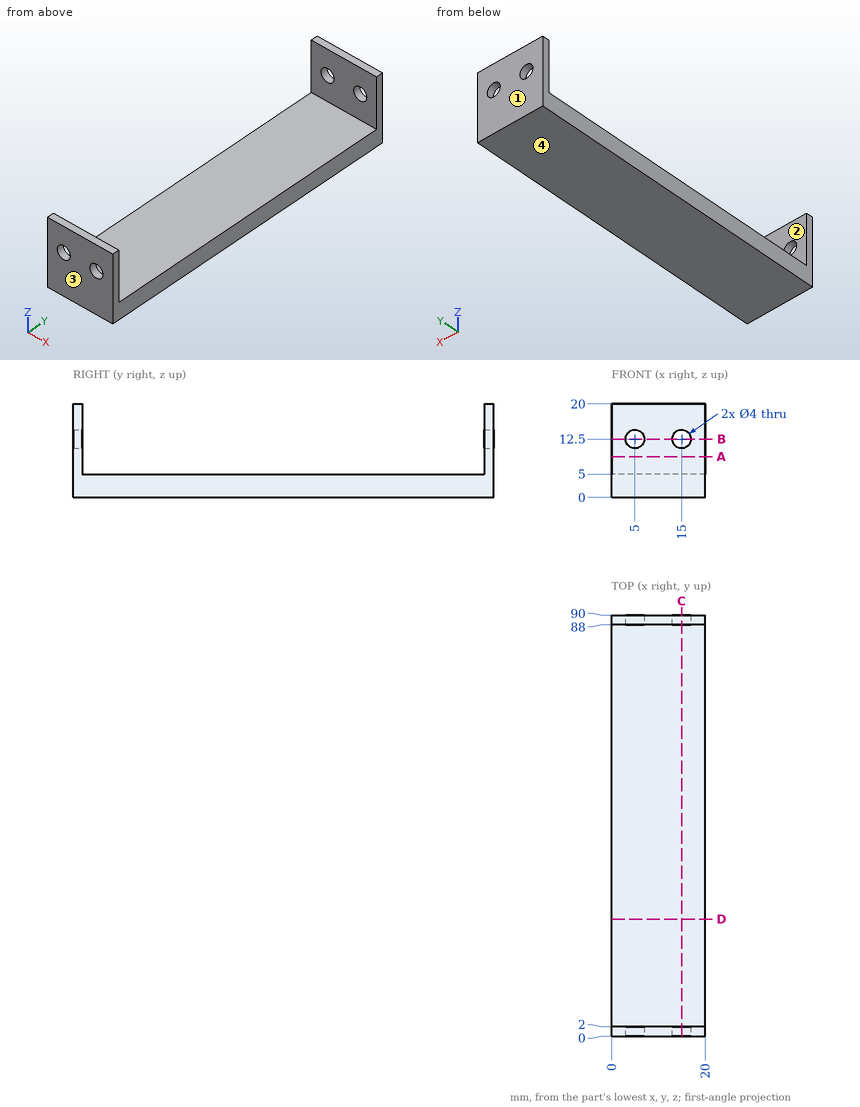
Job drawing, mm, ordinate dimensions from the low corner. One solid piece. Give positions to 0.01 mm unless a question says otherwise; leave off trailing zeros. Write each loop counter-clockwise with the first axis right and the second up, starting at its lowest first coordinate (ties: lowest second). Pieces come first, ordered by that corner, then holes. Notation, with made-up numbers: M 64,11.25 L 103,11.25 A20 cw 103,42.25 Z; hole C 56.5,26 d4. An arc over 180 degrees is marked long. One line per item, written item: value. Start each with the question number.
Q1. Probe probe 1 along X at (y, z) = (0.6, 12.5); probe 2 along Z at (x, y) = (15, 1); probe 3 along Y at (x, z) = (12, 7). List the from-to ranges inside material, lowest first. Write a range as [from, to].
Q2. Drop flat-ended pins along their axis: pin 1 Ø12 at (x, z) = (3, 2.5) entering from -Y; pin 2 Ø3 at (x, z) = (5, 12.5) entering from -Y; pin 3 Ø6 at (x, y) = (5, 27) entering from +Z. Give the stop position or say it passes through.
Q3. Saw through at D-D, the plane y = 25. Write the cut outline in (x, z).
Q4. Saw through at B-B, the plane z = 12.5. Write the cut outline in (x, y), plus the area to 3 significant figures.
Q5. Two-plate mould, pull along Y, no slides. Class the marked faces 1, 2, 3 and 4: +Y half, -Y half, draft (parallel to the pull), parting line (faces both ways), or undercut.
Q6. Saw through at C-C, the plane x = 15. Write the cut outline in (y, z), plus the area to 3 significant figures.
Q7. Saw through at A-A, the plane z = 8.75. Write the cut outline in (x, y), plus the area to 3 significant figures.
Output values:
1. probe 1: x = [0, 3], [7, 13], [17, 20]
1. probe 2: z = [0, 10.5], [14.5, 20]
1. probe 3: y = [0, 2], [88, 90]
2. pin 1: stops at y = 0
2. pin 2: passes through
2. pin 3: stops at z = 5
3. outline: M 0,0 L 20,0 L 20,5 L 0,5 Z
4. outline: M 0,0 L 3,0 L 3,2 L 0,2 Z; M 0,88 L 3,88 L 3,90 L 0,90 Z; M 7,0 L 13,0 L 13,2 L 7,2 Z; M 7,88 L 13,88 L 13,90 L 7,90 Z; M 17,0 L 20,0 L 20,2 L 17,2 Z; M 17,88 L 20,88 L 20,90 L 17,90 Z
4. area: 48.0 mm²
5. face 1: +Y half
5. face 2: undercut
5. face 3: -Y half
5. face 4: draft
6. outline: M 0,0 L 90,0 L 90,10.5 L 88,10.5 L 88,5 L 2,5 L 2,10.5 L 0,10.5 Z; M 0,14.5 L 2,14.5 L 2,20 L 0,20 Z; M 88,14.5 L 90,14.5 L 90,20 L 88,20 Z
6. area: 494 mm²
7. outline: M 0,0 L 20,0 L 20,2 L 0,2 Z; M 0,88 L 20,88 L 20,90 L 0,90 Z
7. area: 80.0 mm²
